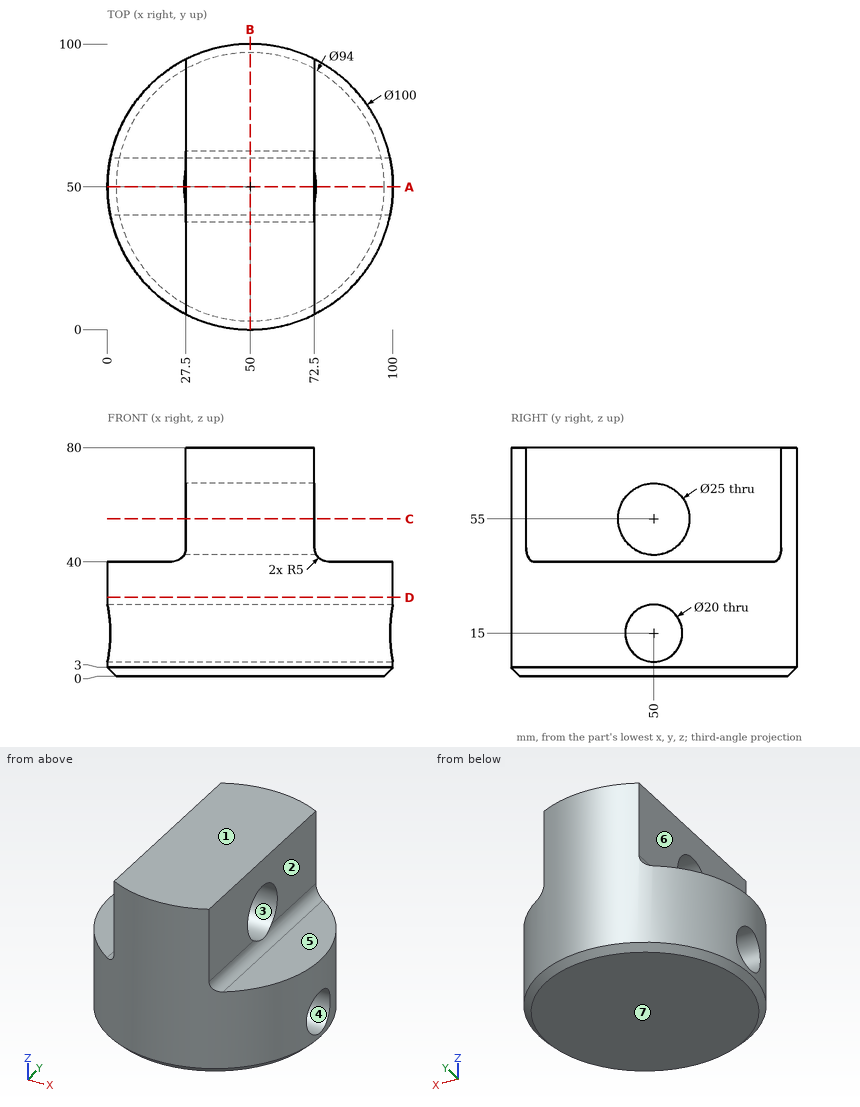
Could you check a few things on this drawing? It's one solid part, dimensions in mm from its lowest x, y, z. A direction names the side the tool comes from. Round coordinates to 2 decimals unless told otherwise and drop trailing zeros. Loops run counter-clockwise (first coordinate to the right, second up) from the corner with the lowest first, then second, coordinate; pieces in that order, holes last. Notation, with made-up numbers: (19, -31) -> (33, -31) arc R30 cw to (33, 5) -> close; hole circle Ø4 at (47.25, 72.5). An arc over 180 degrees is marked (long way). One line per item, written item: value. Start each with the question number.
1. If we section it at A-A, the plane y = 50: Write out the boundary of the cut face in (x, z).
2. If we mould it in two halves opening along Z, with no side actions, what happens to the marked faces 1, 2, 3 and 4? For each: pulls with the +Z half, pulls with the -Z half, needs draft (parallel to the pull), parting line crosses it, or undercut.
3. If we section it at C-C, the plane z = 55: Write out the boundary of the cut face in (x, y).
4. If we section it at D-D, the plane z = 27.5: Write out the boundary of the cut face in (x, y).
5. If I drill on probe 1 along Z at (x, y) = (35.5, 54); probe 2 along X at (y, z) = (64, 54); probe 3 along Z at (x, y) = (28, 47.5), over which ranges is the centre line in solid material (lowest first)?
6. For the marked faces 5, 6 and 7, which set-ups out of +Z, -Z, +X, -X, +Y, -Y let a thin tool reach every point of the face, with its end or its side?
7. For pin 1 (18 mm diameter, centred on x = 8.5, y = 49, fed in from +Z); pin 2 (5 mm diameter, centred on x = 53, z = 48.5, fed in from +Y); pin 3 (1.5 mm diameter, centred on x = 73, z = 30, fed in from +Y), each with a flat end and sliding along its axis, tell me the tip position at first contact or that it passes through.
8. If we section it at B-B, the plane x = 50: Write out the boundary of the cut face in (y, z), then the cut area to 3 significant figures.
Calculated:
1. outline: (0, 3) -> (3, 0) -> (97, 0) -> (100, 3) -> (100, 5) -> (0, 5) -> close; (0, 25) -> (100, 25) -> (100, 40) -> (77.5, 40) arc R5 cw to (73.17, 42.5) -> (26.83, 42.5) arc R5 cw to (22.5, 40) -> (0, 40) -> close; (27.5, 67.5) -> (72.5, 67.5) -> (72.5, 80) -> (27.5, 80) -> close
2. face 1: pulls with the +Z half
2. face 2: needs draft
2. face 3: undercut
2. face 4: undercut
3. outline: (27.5, 5.35) arc R50 ccw to (72.5, 5.35) -> (72.5, 37.5) -> (27.5, 37.5) -> close; (27.5, 62.5) -> (72.5, 62.5) -> (72.5, 94.65) arc R50 ccw to (27.5, 94.65) -> close
4. outline: circle Ø100 at (50, 50)
5. probe 1: z = 0 to 5.83, 24.17 to 43.16, 66.84 to 80
5. probe 2: x = 27.5 to 72.5
5. probe 3: z = 0 to 5.32, 24.68 to 42.75, 67.25 to 80
6. face 5: +Z, +X, +Y, -Y
6. face 6: +Z, -X, +Y, -Y
6. face 7: -Z, +X, -X, +Y, -Y
7. pin 1: stops at z = 40
7. pin 2: stops at y = 100
7. pin 3: stops at y = 94.78
8. outline: (0, 3) -> (3, 0) -> (97, 0) -> (100, 3) -> (100, 80) -> (0, 80) -> close; hole circle Ø25 at (50, 55); hole circle Ø20 at (50, 15)
8. area: 7,190 mm²
